Input: part model. Units: mm. Frame: model coordinates. Face numbers are marked on the shaded views. A direction names the side the tool comes from. Round coordinates to 2 decimals unless told otherwise and drop trailing zeros. Loops run counter-clockwise (first coordinate to the right, second up) from the corner with the lowest first, then second, coordinate; pieces in that order, holes last. Notation, with made-up numbers: (56, 39.25) -> (97, 39.25) arc R9 cw to (97, 50.25) -> close; hole circle Ø9 at (-34, -40). An arc over 180 degrees is marked (long way). Answer in a Markdown table with one row per item. Add a question column.
Q1. Ray query, L1, parallel to X at y = 4.75, z = 13.97; L2, parallel to X at y = 1.75, z = 13.97; L3, parallel to X at y = 2.25, z = 2. Return the intervals inside material, ascending. Write a range as from..to.
Q2. Section D-D, the plane y = 8.75. Output: boundary loops of the cut face in (x, z).
Q3. Reachability of the marked faces 1, 2, 3 and 4 from +Z, -Z, +X, -X, +Y, -Y: full face, straight path, thin tool, end or side. Return the list, or none.
Q4. Section C-C, the plane z = 3. Output: boundary loops of the cut face in (x, y), and give its area (3 significant figures).
Q5. Mould query, pull axis X, two halves, no side actions, for the marked faces 5, 6, 7 and 8. Classes: pulls with the +X half, pulls with the -X half, needs draft (parallel to the pull), parting line crosses it, or undercut.
Q6. Section B-B, the plane x = -1.5. Output: boundary loops of the cut face in (y, z).
Q7. Pin query (flat end, axial travel): pin 1 (2.5 mm diameter, centred on x = -1, z = 14.5, fed in from -Y); pin 2 (5 mm diameter, centred on x = 0.5, y = 1.5, fed in from -Z); pin 3 (2 mm diameter, centred on x = -0.5, z = 9.5, fed in from -Y). Return the tip coordinate at first contact, or that it passes through.
Q8. Section A-A, the plane z = 13.97. Output: boundary loops of the cut face in (x, y).
Autodesk Inventor part; units mm, degrees
ref_plane "YZ Plane" through (0, 0, 0) normal (1, 0, 0) x (0, 1, 0)
ref_plane "XZ Plane" through (0, 0, 0) normal (0, 1, 0) x (-1, 0, 0)
ref_plane "XY Plane" through (0, 0, 0) normal (0, 0, 1) x (1, 0, 0)
sketch "XT60" plane through (0, 0, 0) normal (0, 0, 1) x (1, 0, 0)
  line L0 (-7.6835, 4.0132) -> (7.6835, 4.0132) construction
  line L1 (7.6835, 4.0132) -> (7.6835, -4.0132)
  line L2 (7.6835, -4.0132) -> (-7.6835, -4.0132) construction
  line L3 (-7.6835, -4.0132) -> (-7.6835, 4.0132) construction
  line L4 (-7.6835, 4.0132) -> (7.6835, -4.0132) construction
  line L5 (7.6835, 4.0132) -> (-7.6835, -4.0132) construction
  line L6 (-7.6835, 2.2171) -> (-5.8874, 4.0132)
  line L7 (-7.6835, 2.2171) -> (-5.1435, 2.2171) construction
  line L8 (-10.7569, 0) -> (10.7569, 0)
  line L9 (-7.6835, -2.2171) -> (-5.8874, -4.0132)
  line L10 (-7.6835, -2.2171) -> (-5.1435, -2.2171) construction
  line L11 (-7.6835, -2.2171) -> (-7.6835, 2.2171)
  line L12 (-5.8874, 4.0132) -> (7.6835, 4.0132)
  line L13 (7.6835, -4.0132) -> (-5.8874, -4.0132)
  point P0 (0, 0)
  dimension "d0" = 15.367
  dimension "d1" = 8.0264
  dimension "d2" = 2.54
  dimension "d3" = 45
  dimension "d4" = 2.54
  dimension "d5" = 45
sketch "Sketch2" plane through (0, 0, 0) normal (0, 0, 1) x (1, 0, 0)
  line L0 (-7.6835, 2.2171) -> (-5.8874, 4.0132)
  line L1 (-5.8874, 4.0132) -> (7.6835, 4.0132)
  line L2 (-7.6835, -2.2171) -> (-7.6835, 2.2171)
  line L3 (-7.6835, -2.2171) -> (-5.8874, -4.0132)
  line L4 (7.6835, -4.0132) -> (-5.8874, -4.0132)
  line L5 (7.6835, 4.0132) -> (7.6835, -4.0132)
  line L6 (8.1915, 4.5212) -> (-6.0979, 4.5212)
  line L7 (-6.0979, 4.5212) -> (-8.1915, 2.4276)
  line L8 (-8.1915, 2.4276) -> (-8.1915, -2.4276)
  line L9 (-8.1915, -2.4276) -> (-6.0979, -4.5212)
  line L10 (-6.0979, -4.5212) -> (8.1915, -4.5212)
  line L11 (8.1915, -4.5212) -> (8.1915, 4.5212)
  line L12 (7.4295, 3.7592) -> (-5.7822, 3.7592)
  line L13 (-5.7822, 3.7592) -> (-7.4295, 2.1119)
  line L14 (-7.4295, 2.1119) -> (-7.4295, -2.1119)
  line L15 (-7.4295, -2.1119) -> (-5.7822, -3.7592)
  line L16 (-5.7822, -3.7592) -> (7.4295, -3.7592)
  line L17 (7.4295, -3.7592) -> (7.4295, 3.7592)
  line L18 (-19.05, 6.35) -> (19.05, 6.35)
  line L19 (19.05, 6.35) -> (19.05, 0)
  line L20 (19.05, 0) -> (-19.05, 0)
  line L21 (-19.05, 0) -> (-19.05, 6.35)
  line L22 (-5.9055, -2.413) -> (5.9055, -2.413)
  line L23 (5.9055, -2.413) -> (5.9055, 2.413)
  line L24 (5.9055, 2.413) -> (-5.9055, 2.413)
  line L25 (-5.9055, 2.413) -> (-5.9055, -2.413)
  line L26 (-5.9055, -2.413) -> (5.9055, 2.413) construction
  line L27 (5.9055, -2.413) -> (-5.9055, 2.413) construction
  line L28 (-19.05, 6.35) -> (19.05, 6.35)
  line L29 (19.05, 6.35) -> (19.05, 12.7)
  line L30 (19.05, 12.7) -> (-19.05, 12.7)
  line L31 (-19.05, 12.7) -> (-19.05, 6.35)
  point P0 (0, 0)
  dimension "d6" = 0.254
  dimension "d7" = 0.508
  dimension "d8" = 38.1
  dimension "d9" = 6.35
  dimension "d25" = 11.811
  dimension "d26" = 4.826
  dimension "d29" = 6.35
extrude "Extrusion1" add sketch "Sketch2" along normal blind 27.94 contours L2 L20 L8 L7 L6 L11 L5 L1 L0 | L0 L1 L5 L20 L17 L12 L13 L14 L2 | L14 L13 L12 L17 L20 L23 L24 L25 | L20 L21 L18 L19 L11 L6 L7 L8 | L25 L24 L23 L20
extrude "Extrusion2" cut sketch "Sketch2" along normal blind 18.3896 contours L20 L25 L22 L23 L17 L16 L15 L14 | L14 L13 L12 L17 L20 L23 L24 L25 | L25 L24 L23 L20 | L20 L23 L22 L25
extrude "Extrusion3" cut sketch "Sketch2" along normal blind 10.6172 contours L2 L20 L8 L7 L6 L11 L5 L1 L0 | L0 L1 L5 L20 L17 L12 L13 L14 L2 | L20 L14 L15 L16 L17 L5 L4 L3 L2 | L2 L3 L4 L5 L20 L11 L10 L9 L8 | L20 L25 L22 L23 L17 L16 L15 L14 | L14 L13 L12 L17 L20 L23 L24 L25 | L25 L24 L23 L20 | L20 L23 L22 L25
sketch "Sketch3" plane through (0, 0, 0) normal (0, 1, 0) x (-1, 0, 0)
  point P0 (-16.002, 13.97)
  point P1 (0, 0)
  dimension "d16" = 16.002
  dimension "d17" = 13.97
hole "Hole1" at (16.002, 0, 13.97) direction (0, 1, 0) diameter 3.2766 end through all
mirror "Mirror1" about plane through (0, 0, 0) normal (1, 0, 0) of "Hole1"
extrude "Extrusion4" cut sketch "Sketch2" along normal through all contours L25 L24 L23 L20 | L20 L23 L22 L25
extrude "Extrusion5" add sketch "Sketch2" along normal blind 6.35 contours L31 L30 L29 L18
properties part number "xt-60 holder"
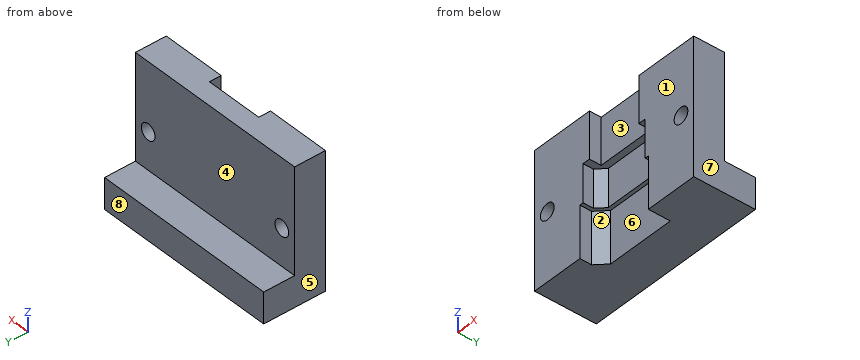
Answer block:
| question | item | result |
|---|---|---|
| 1 | L1 | -19.05..-17.64, -14.36..14.36, 17.64..19.05 |
| 1 | L2 | -19.05..-17.64, -14.36..-7.43, 7.43..14.36, 17.64..19.05 |
| 1 | L3 | -19.05..-8.19, 8.19..19.05 |
| 2 | outline | (-19.05, 0) -> (19.05, 0) -> (19.05, 6.35) -> (-19.05, 6.35) -> close |
| 3 | face 1 | +Z, -Z, +X, -X, -Y |
| 3 | face 2 | -Z, -Y |
| 3 | face 3 | +Z, -Z, -Y |
| 3 | face 4 | +Z, +X, -X, +Y |
| 4 | outline | (-19.05, 0) -> (-8.19, 0) -> (-8.19, 2.43) -> (-6.1, 4.52) -> (8.19, 4.52) -> (8.19, 0) -> (19.05, 0) -> (19.05, 12.7) -> (-19.05, 12.7) -> close |
| 4 | area | 412 mm^2 |
| 5 | face 5 | pulls with the -X half |
| 5 | face 6 | undercut |
| 5 | face 7 | pulls with the +X half |
| 5 | face 8 | needs draft |
| 6 | outline | (2.41, 18.39) -> (3.76, 18.39) -> (3.76, 10.62) -> (4.52, 10.62) -> (4.52, 0) -> (12.7, 0) -> (12.7, 6.35) -> (6.35, 6.35) -> (6.35, 27.94) -> (2.41, 27.94) -> close |
| 7 | pin 1 | y = 3.76 |
| 7 | pin 2 | z = 10.62 |
| 7 | pin 3 | y = 4.52 |
| 8 | outline | (-19.05, 0) -> (-17.64, 0) -> (-17.64, 6.35) -> (-19.05, 6.35) -> close; (-14.36, 0) -> (-7.43, 0) -> (-7.43, 2.11) -> (-5.78, 3.76) -> (7.43, 3.76) -> (7.43, 0) -> (14.36, 0) -> (14.36, 6.35) -> (-14.36, 6.35) -> close; (17.64, 0) -> (19.05, 0) -> (19.05, 6.35) -> (17.64, 6.35) -> close |
